```python
from build123d import *

# Parameters (mm, degrees)
CUT_EXTRUDE_1_DEPTH      = 1636.725546456
CUT_EXTRUDE_1_DEPTH_BACK = 1636.725546456
SKETCH_3_OUTSIDE_W       = 2264.278
SKETCH_3_OUTSIDE_H       = 2264.278
CUT_EXTRUDE_5_DEPTH      = 10
HOLE_WIZARD_M5_1_D       = 4.2


with BuildPart() as part:
    # 草图2 → 旋转1 (revolve)
    with BuildSketch(Plane.XY):
        Polygon((-422.349891291, 6.062538723), (-42.349891291, 6.062538723), (337.650108709, 320.562538723), (357.650108709, 320.562538723), (357.650108709, 317.115170302), (-42.349891291, -13.937461277), (-422.349891291, -13.937461277), align=None)
    revolve(axis=Axis((457.650108709, 481.315085819, 0), (0, -1, 0)))

    # 草图3 outside → 切除-拉伸1 (cut, two sides: drawn at the far end of the back side and taken through both)
    with BuildSketch(Plane(origin=(0, 320.562538723, 0), x_dir=(1, 0, 0), z_dir=(0, 1, 0)).offset(-CUT_EXTRUDE_1_DEPTH_BACK)):
        with Locations((457.65, 0)):
            Rectangle(SKETCH_3_OUTSIDE_W, SKETCH_3_OUTSIDE_H)
        Polygon((457.650108709, 0), (1205.950605112, 776.341843522), (29.226896752, 1910.562473831), (-719.073599651, 1134.220630309), align=None, mode=Mode.SUBTRACT)
    extrude(amount=CUT_EXTRUDE_1_DEPTH + CUT_EXTRUDE_1_DEPTH_BACK, mode=Mode.SUBTRACT)

    # 草图7 → 切除-拉伸5 (cut)
    with BuildSketch(Plane.XZ.offset(13.937461277)):
        Polygon((395.372807922, -667.072096819), (405.372807922, -667.072096819), (406.034922879, -631.072096819), (396.034922879, -631.072096819), (395.7038654, -649.072096819), align=None)
        Polygon((495.686956256, -650.910994037), (496.018013734, -632.910994037), (486.018013734, -632.910994037), (486.018013734, -668.907950391), (495.355954757, -668.907950391), align=None)
    extrude(amount=-CUT_EXTRUDE_5_DEPTH, mode=Mode.SUBTRACT)

    # M5 螺纹孔1 (through all)
    with Locations(Plane(origin=(-145.171244311, 6.062538723, -619.24250439), x_dir=(1, 0, 0), z_dir=(0, 1, 0))):
        with Locations((0, 0), (35.99950912, -34.699212428)):
            hole_wizard_m5_1 = Hole(HOLE_WIZARD_M5_1_D / 2)

    # 镜向1: M5 螺纹孔1 across plane
    add(hole_wizard_m5_1.mirror(Plane(origin=(457.495352358, 0, -8.41429209), x_dir=(0.018388972176112385, 0, 0.9998309085551947), z_dir=(-0.9998309085551947, 0, 0.018388972176112385))), mode=Mode.SUBTRACT)


solid = part.part
```
Could you check a few things on this model? Use its own coordinates, in mm. Coordinates: 2 decimals unless noted, no trailing zeros. Write each loop counter-clockwise with the first axis right and the second up, starting at its lowest first coordinate (ties: lowest second). Pieces come first, ordered by that corner, then holes. Notation, with made-up numbers: (49.5, 24) -> (80.5, 24) arc R9 cw to (80.5, 41) -> close; hole circle Ø2 at (48.25, -3). An arc over 180 degrees is marked (long way). Write item = value, one per line. Start each with the question number.
(1) I want a section at A-A (z = -811). Please give me the cut outline in (x, y), plus the area to 3 significant figures.
(2) Will these pins go through, and if not, where does the flat tip stop? pin 1 (3 mm diameter, centred on x = 398, y = -9.5, fed in from +Z); pin 2 (8 mm diameter, centred on x = 318.5, y = 159, fed in from +Z); pin 3 (1 mm diameter, centred on y = 152, z = -240, fed in from -X); pin 4 (3.5 mm diameter, centred on x = 1037.29, z = -640.99, fed in from +Y).
(3) We'd pull the mould along X, two halves only. Please class faces 1 (the face through (124.34, 28.64, -321.27)), 2 (the face through (454.712, 318.815, -99.957)), 3 (the face through (431.79, -3.8, -879.62)), 4 (the face through (448.75, 149.27, -302.67)): released by +X, released by -X, zero draft, split by the parting line, or undercut.
(4) I need wall thicknesses on line 1 (Y direction, x = 191, z = -430); line 2 (X direction, y = 19.5, z = -387.5); line 3 (X direction, y = 113, z = -291). Which ranges of each line are inside material? Lowest first, please. Write a range as [from, to].
(5) I want a section at B-B (y = 156.5). Please give me the cut outline in (x, z), plus the area to 3 significant figures.
Result set:
q1.outline = (116.07, -13.94) -> (799.23, -13.94) -> (799.23, 6.06) -> (116.07, 6.06) -> close
q1.area = 13,700 mm2
q2.pin_1 = -489.19
q2.pin_2 = -249.67
q2.pin_3 = 239.43
q2.pin_4 = through
q3.face_1 = released by -X
q3.face_2 = undercut
q3.face_3 = split by the parting line
q3.face_4 = undercut
q4.line_1 = [-13.94, 6.06]
q4.line_2 = [168.04, 210.52], [704.78, 747.26]
q4.line_3 = [227.86, 269.32], [645.98, 687.44]
q5.outline = (228.53, -220.85) arc R318.23 ccw to (678.5, -229.12) -> (661.73, -211.72) arc R294.07 cw to (245.93, -204.08) -> close
q5.area = 11,600 mm2
